```python
from build123d import *

# Parameters (mm, degrees)
SKETCH24_R          = 5.4
SKETCH24_W          = 4
SKETCH24_H          = 3
BOSS_EXTRUDE1_DEPTH = 20
SKETCH28_W          = 7
SKETCH28_H          = 32.25
BOSS_EXTRUDE2_DEPTH = 20
SKETCH25_R          = 5.4
CUT_EXTRUDE1_DEPTH  = 20
SKETCH26_R          = 4.2
CUT_EXTRUDE2_DEPTH  = 18
SKETCH27_R          = 10.75
CUT_EXTRUDE3_DEPTH  = 2
FILLET4_R           = 3
FILLET6_R           = 3
SKETCH31_R          = 3
CUT_EXTRUDE5_DEPTH  = 7
SKETCH32_W          = 3
SKETCH32_H          = 5.8
BOSS_EXTRUDE3_DEPTH = 3


with BuildPart() as part:
    # Sketch24 → Boss-Extrude1 (new body)
    with BuildSketch(Plane(origin=(0, 0, 0), x_dir=(0, 0, -1), z_dir=(1, 0, 0))):
        Polygon((10, -9.157855987), (10, 46.842144013), (-10, 46.842144013), (-10, -9.157855987), (-2.9, -9.157855987), (-2.9, -12.157855987), (2.9, -12.157855987), (2.9, -9.157855987), align=None)
        with Locations((0, 24.842144013)):
            Circle(SKETCH24_R, mode=Mode.SUBTRACT)
        with Locations((0, 2.842144013)):
            Circle(SKETCH24_R, mode=Mode.SUBTRACT)
        with Locations((-0.353280434, 37.342144013)):
            Rectangle(SKETCH24_W, SKETCH24_H, mode=Mode.SUBTRACT)
    extrude(amount=BOSS_EXTRUDE1_DEPTH)

    # Sketch28 → Boss-Extrude2 (add)
    with BuildSketch(Plane(origin=(20, 0, 0), x_dir=(0, 0, -1), z_dir=(1, 0, 0))):
        with Locations((-13.5, -13.032855987)):
            Rectangle(SKETCH28_W, SKETCH28_H)
    extrude(amount=-BOSS_EXTRUDE2_DEPTH)

    # Sketch25 → Cut-Extrude1 (cut)
    with BuildSketch(Plane.XY.offset(10)):
        with Locations((10, 13.842144013)):
            Circle(SKETCH25_R)
    extrude(amount=-CUT_EXTRUDE1_DEPTH, mode=Mode.SUBTRACT)

    # Sketch26 → Cut-Extrude2 (cut)
    with BuildSketch(Plane.XY.offset(10)):
        with Locations((10, 44.842144013)):
            Circle(SKETCH26_R)
    extrude(amount=-CUT_EXTRUDE2_DEPTH, mode=Mode.SUBTRACT)

    # Sketch27 → Cut-Extrude3 (cut)
    with BuildSketch(Plane(origin=(0, 0, -10), x_dir=(-1, 0, 0), z_dir=(0, 0, -1))):
        with Locations((-10, 13.842144013)):
            Circle(SKETCH27_R)
    extrude(amount=-CUT_EXTRUDE3_DEPTH, mode=Mode.SUBTRACT)

    # Fillet4
    fillet4_edges = [part.edges().sort_by_distance(p)[0] for p in [
        (10, 3.092144013, 17),
    ]]
    fillet(fillet4_edges, radius=FILLET4_R)

    # Fillet6
    fillet6_edges = [part.edges().sort_by_distance(p)[0] for p in [
        (10, 3.092144013, 10),
    ]]
    fillet(fillet6_edges, radius=FILLET6_R)

    # Sketch31 → Cut-Extrude5 (cut)
    with BuildSketch(Plane.XY.offset(17)):
        with Locations((10, -19.157855987)):
            Circle(SKETCH31_R)
    extrude(amount=-CUT_EXTRUDE5_DEPTH, mode=Mode.SUBTRACT)

    # Sketch32 → Boss-Extrude3 (add)
    with BuildSketch(Plane(origin=(0, 0, 10), x_dir=(-1, 0, 0), z_dir=(0, 0, -1))):
        with Locations((-1.5, -19.157855987)):
            Rectangle(SKETCH32_W, SKETCH32_H)
        with Locations((-18.5, -19.157855987)):
            Rectangle(SKETCH32_W, SKETCH32_H)
    extrude(amount=BOSS_EXTRUDE3_DEPTH)


solid = part.part
```
Part model, mm, in its own coordinate system. A direction names the side the tool comes from. Round coordinates to 2 decimals unless told otherwise and drop trailing zeros. Loops run counter-clockwise (first coordinate to the right, second up) from the corner with the lowest first, then second, coordinate; pieces in that order, holes last.
Item 1: Cut at B-B, the plane x = 10. State how many separate pieces and enclosed holes the cut face has, then the cut area to 3 significant figures.
Item 2: Cut at D-D, the plane x = 17.75. Give the cut face in (y, z).
Item 3: Cut at C-C, the plane y = 27. Give the cut face in (x, z), then the cut area to 3 significant figures.
Item 4: Mould opens along X. For faces 4 (the face through (10, 35.842, 0)), 5 (the face through (9.82, 24.59, -9.01)) say: +X half, -X half, draft (parallel to the pull), parting line (faces both ways), or undercut.
Item 5: Drill centre lines: line 1 (Y direction, x = 10, z = -4); line 2 (Y direction, x = 1, z = 4.25); line 3 (Y direction, x = 18.75, z = -1). Where is each one in solid material? Low to high.
Item 6: 3-axis set-ups, long thin cutter, end or side, ignore diameter. For faces 1 (the face through (15, 19, -8)), 2 (the face through (17, -19, 9)), 3 (the face through (10, -11, 2.9)): which of +Z, -Z, +X, -X, +Y, -Y reach the whole face in a straight line?
Item 7: Cut at A-A, the plane z = 0. Give the cut face in (x, y).
Item 8: Drop flat-ended pins along their axis: P1, Ø9.5, axis at y = 2.84, z = 0, coming from the +X side; P2, Ø3, axis at x = 11, z = 0, coming from the -Y side; P3, Ø2.5, axis at x = 2, z = 8.5, coming from the -Y side; P4, Ø0.9, axis at x = 1, y = -18, coming from the -Z side. Give the stop position or say it passes through.
A:
1. separate pieces: 3
1. enclosed holes: 3
1. area: 777 mm2
2. outline: (-29.16, 10) - (-22.06, 10) - (-22.06, 7) - (-16.26, 7) - (-16.26, 10) - (-9.16, 10) - (-9.16, 2.9) - (-12.16, 2.9) - (-12.16, -2.9) - (-9.16, -2.9) - (-9.16, -10) - (6.39, -10) - (6.39, -8) - (21.29, -8) - (21.29, -10) - (46.84, -10) - (46.84, 10) - (6.09, 10) arc R3 cw to (3.09, 13) - (3.09, 14) arc R3 ccw to (0.09, 17) - (-29.16, 17) - close; hole circle Ø10.8 at (2.84, 0); hole circle Ø10.8 at (24.84, 0); hole (35.84, -1.65) - (38.84, -1.65) - (38.84, 2.35) - (35.84, 2.35) - close
3. outline: (0, -10) - (20, -10) - (20, -4.95) - (0, -4.95) - close; (0, 4.95) - (20, 4.95) - (20, 10) - (0, 10) - close
3. area: 202 mm2
4. face 4: draft
4. face 5: undercut
5. line 1: y = -9.16 to -0.79, 6.47 to 8.44, 19.24 to 21.21, 28.47 to 40.64
5. line 2: y = -9.16 to -0.49, 6.17 to 21.51, 28.17 to 46.84
5. line 3: y = -12.16 to -2.46, 8.15 to 19.54, 30.15 to 35.84, 38.84 to 46.84
6. face 1: -Z
6. face 2: -Z, -Y
6. face 3: +X, -X, -Y
7. outline: (0, -12.16) - (20, -12.16) - (20, -2.56) - (0, -2.56) - close; (0, 8.24) - (20, 8.24) - (20, 19.44) - (0, 19.44) - close; (0, 30.24) - (20, 30.24) - (20, 35.84) - (0, 35.84) - close; (0, 38.84) - (20, 38.84) - (20, 46.84) - (13.69, 46.84) arc R4.2 cw (long way) to (6.31, 46.84) - (0, 46.84) - close; hole circle Ø10.8 at (10, 13.84)
8. P1: passes through
8. P2: stops at y = -12.16
8. P3: stops at y = -22.06
8. P4: stops at z = 7
